Can you work these out from the drawing? Everything is in mm from the part's minimum corner. A direction names the side the tool comes from. Round coordinates to 2 decimals unless told otherwise and drop trailing zeros. Loops run counter-clockwise (first coordinate to the right, second up) from the corner with the lowest first, then second, coordinate; pieces in that order, holes last. Notation, with made-up numbers: M 28.25,6 L 58.25,6 A29 cw 58.25,34 Z; hole C 83,-7.75 d6. An arc over 180 degrees is marked long. Answer in a Markdown table with one row per item.
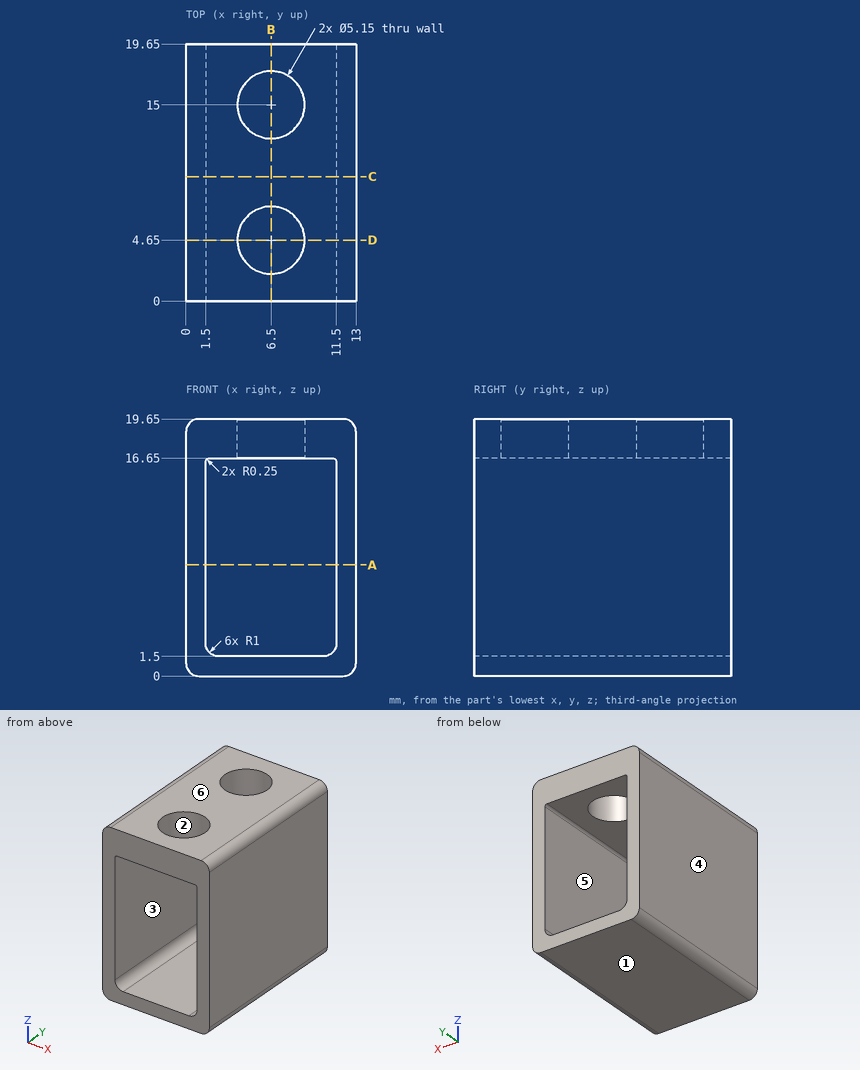
1) If we mould it in two halves opening along Z, with no side actions, what happens to the marked faces 4, 5 and 6? For each: released by +Z, released by -Z, zero draft, split by the parting line, or undercut.
Computed:
| item | result |
|---|---|
| face 4 | zero draft |
| face 5 | undercut |
| face 6 | released by +Z |
2) I need wall thicknesses on line 1 (Y direction, x = 6.5, z = 18.4) (3 decimals); line 2 (X direction, y = 7, z = 9); line 3 (Z direction, x = 4.5, y = 11). Which ranges of each line are inside material? Lowest first, please.
Computed:
| item | result |
|---|---|
| line 1 | y = 0 to 2.075, 7.225 to 12.425, 17.575 to 19.65 |
| line 2 | x = 0 to 1.5, 11.5 to 13 |
| line 3 | z = 0 to 1.5, 16.65 to 19.65 |
3) I want a section at D-D, the plane y = 4.65. Please give me the cut outline in (x, z) (3 decimals).
Computed:
| item | result |
|---|---|
| outline | M 0,1 A1 ccw 1,0 L 12,0 A1 ccw 13,1 L 13,18.65 A1 ccw 12,19.65 L 9.075,19.65 L 9.075,16.65 L 11.25,16.65 A0.25 cw 11.5,16.4 L 11.5,2.5 A1 cw 10.5,1.5 L 2.5,1.5 A1 cw 1.5,2.5 L 1.5,16.4 A0.25 cw 1.75,16.65 L 3.925,16.65 L 3.925,19.65 L 1,19.65 A1 ccw 0,18.65 Z |
4) I want a section at A-A, the plane z = 8.5. Please give me the cut outline in (x, y).
Computed:
| item | result |
|---|---|
| outline | M 0,0 L 1.5,0 L 1.5,19.65 L 0,19.65 Z; M 11.5,0 L 13,0 L 13,19.65 L 11.5,19.65 Z |
5) I want a section at C-C, the plane y = 9.5. Please give me the cut outline in (x, z), plus the area to 3 significant figures.
Computed:
| item | result |
|---|---|
| outline | M 0,1 A1 ccw 1,0 L 12,0 A1 ccw 13,1 L 13,18.65 A1 ccw 12,19.65 L 1,19.65 A1 ccw 0,18.65 Z; hole M 1.5,2.5 A1 ccw 2.5,1.5 L 10.5,1.5 A1 ccw 11.5,2.5 L 11.5,16.4 A0.25 ccw 11.25,16.65 L 1.75,16.65 A0.25 ccw 1.5,16.4 Z |
| area | 104 mm² |
6) I want a section at B-B, the plane x = 6.5. Please give me the cut outline in (y, z) (3 decimals), plus the area to 3 significant figures.
Computed:
| item | result |
|---|---|
| outline | M 0,0 L 19.65,0 L 19.65,1.5 L 0,1.5 Z; M 0,16.65 L 2.075,16.65 L 2.075,19.65 L 0,19.65 Z; M 7.225,16.65 L 12.425,16.65 L 12.425,19.65 L 7.225,19.65 Z; M 17.575,16.65 L 19.65,16.65 L 19.65,19.65 L 17.575,19.65 Z |
| area | 57.5 mm² |
7) Will this pin go through, and if not, where does the flat tip stop? P1, Ø3, axis at x = 6.5, y = 11, coming from the -Z side.
Computed:
| item | result |
|---|---|
| P1 | stops at z = 0 |
8) Which directions (+Z, -Z, +X, -X, +Y, -Y) give clear straight access to the entire face, cutting with the end or side of a thin tool? Please do the marked faces 1, 2 and 3.
Computed:
| item | result |
|---|---|
| face 1 | -Z, +X, -X, +Y, -Y |
| face 2 | +Z |
| face 3 | +Y, -Y |
